Design review of the part built by this model. Coordinates are the model's own, in mm. A direction names the side the tool comes from. Give positions to 0.01 mm unless a question says otherwise; leave off trailing zeros. Loops run counter-clockwise (first coordinate to the right, second up) from the corner with the lowest first, then second, coordinate; pieces in that order, holes last. Notation, with made-up numbers: M 41,49.25 L 90,49.25 A20 cw 90,78.25 Z; hole C 58,85.25 d8. An arc over 180 degrees is marked long. Answer as CSV lines item,"result".
```python
from build123d import *

# Parameters (mm, degrees)
SKETCH1_W           = 38.1
SKETCH1_H           = 10.16
SKETCH1_W_2         = 12.7
SKETCH1_R           = 2.54
BOSS_EXTRUDE1_DEPTH = 50.8
SKETCH2_W           = 63.5
SKETCH2_H           = 50.8
CUT_EXTRUDE1_DEPTH  = 61.761238467


with BuildPart() as part:
    # Sketch1 → Boss-Extrude1 (new body)
    # profile 1 of 3: a face of its own
    with BuildSketch(Plane(origin=(0, 0, 0), x_dir=(1, 0, 0), z_dir=(0, 1, 0))):
        with Locations((0, -1.905)):
            Rectangle(SKETCH1_W, SKETCH1_H)
    # profile 2 of 3: a face of its own
    with BuildSketch(Plane(origin=(0, 0, 0), x_dir=(1, 0, 0), z_dir=(0, 1, 0))):
        with Locations((-25.4, -1.905)):
            Rectangle(SKETCH1_W_2, SKETCH1_H)
        with Locations(Location((-25.4, -1.905, 0), (0, 0, 270))):
            Circle(SKETCH1_R, mode=Mode.SUBTRACT)
    # profile 3 of 3: a face of its own
    with BuildSketch(Plane(origin=(0, 0, 0), x_dir=(1, 0, 0), z_dir=(0, 1, 0))):
        with Locations((25.4, -1.905)):
            Rectangle(SKETCH1_W_2, SKETCH1_H)
        with Locations(Location((25.4, -1.905, 0), (0, 0, 270))):
            Circle(SKETCH1_R, mode=Mode.SUBTRACT)
    extrude(amount=BOSS_EXTRUDE1_DEPTH)

    # Sketch2 → Cut-Extrude1 (cut, through all)
    # profile 1 of 2: a face of its own
    with BuildSketch(Plane.XY.offset(6.985)):
        with Locations((0, 25.4)):
            Rectangle(SKETCH2_W, SKETCH2_H)
        with BuildLine():
            Line((-11.43, 10.16), (-30.48, 10.16))
            Line((-30.48, 10.16), (-30.48, 14.258420741))
            Line((-30.48, 14.258420741), (-18.493061175, 14.258420741))
            ThreePointArc((-18.493061175, 14.258420741), (0, 46.99), (18.493061175, 14.258420741))
            Line((18.493061175, 14.258420741), (30.48, 14.258420741))
            Line((30.48, 14.258420741), (30.48, 10.16))
            Line((30.48, 10.16), (11.43, 10.16))
            ThreePointArc((11.43, 10.16), (0, 44.45), (-11.43, 10.16))
        make_face(mode=Mode.SUBTRACT)
    # profile 2 of 2: a face of its own
    with BuildSketch(Plane.XY.offset(6.985)):
        with Locations((0, 25.4)):
            Rectangle(SKETCH2_W, SKETCH2_H)
        with BuildLine():
            Line((-11.43, 10.16), (-30.48, 10.16))
            Line((-30.48, 10.16), (-30.48, 14.258420741))
            Line((-30.48, 14.258420741), (-18.493061175, 14.258420741))
            ThreePointArc((-18.493061175, 14.258420741), (0, 46.99), (18.493061175, 14.258420741))
            Line((18.493061175, 14.258420741), (30.48, 14.258420741))
            Line((30.48, 14.258420741), (30.48, 10.16))
            Line((30.48, 10.16), (11.43, 10.16))
            ThreePointArc((11.43, 10.16), (0, 44.45), (-11.43, 10.16))
        make_face(mode=Mode.SUBTRACT)
    extrude(amount=-CUT_EXTRUDE1_DEPTH, mode=Mode.SUBTRACT)


solid = part.part
```
1. To check wall thickness, follow L1, parallel to Z at x = 25.4, y = 11.85 (3 decimals); L2, parallel to X at y = 25.4, z = 4.5; L3, parallel to X at y = 13, z = -2.5. State the ranges of each line that lie inside material, in increasing order. Write a range as [from, to].
Answer block:
L1,"[-3.175, -0.635], [4.445, 6.985]"
L2,"[-21.59, -19.05], [19.05, 21.59]"
L3,"[-30.48, -14.46], [14.46, 30.48]"
2. The part is to be moulded in two halves that separate along Y. For faces 3 (the cylindrical face through (-27.88, 12.18, 1.35)), 4 (the flat face through (22, 14.258, 2)), 5 (the flat face through (21, 10.16, 2)), say which applies: pulls with the +Y half, pulls with the -Y half, needs draft (parallel to the pull), parting line crosses it, or undercut.
Answer block:
face 3,"needs draft"
face 4,"undercut"
face 5,"pulls with the -Y half"
3. We need section B-B, the plane x = 25.4. Write out the cut boundary in (y, z) (3 decimals), plus the area to 3 significant figures.
Answer block:
outline,"M 10.16,-3.175 L 14.258,-3.175 L 14.258,-0.635 L 10.16,-0.635 Z; M 10.16,4.445 L 14.258,4.445 L 14.258,6.985 L 10.16,6.985 Z"
area,"20.8 mm²"
4. For faces 1 (the flat face through (30.48, 12, 2)), 2 (the flat face through (-22, 14.258, 2)), list the 3-axis set-ups (+Z, -Z, +X, -X, +Y, -Y) from which the entire face can be reached by the end or side of a thin tool; tool diameter is ignored.
Answer block:
face 1,"+Z, -Z, +X, +Y, -Y"
face 2,"+Z, -Z, -X"
5. We need section C-C, the plane z = 0.5. Write out the cut boundary in (x, y).
Answer block:
outline,"M -30.48,10.16 L -27.52,10.16 L -27.52,14.26 L -30.48,14.26 Z; M -23.28,10.16 L -11.43,10.16 A19.05 cw long 11.43,10.16 L 23.28,10.16 L 23.28,14.26 L 18.49,14.26 A21.59 ccw long -18.49,14.26 L -23.28,14.26 Z; M 27.52,10.16 L 30.48,10.16 L 30.48,14.26 L 27.52,14.26 Z"
6. For P1, Ø5, axis at y = 19, z = -1.5, coming from the -X side; P2, Ø1.5, axis at y = 35, z = 1.5, coming from the -X side; P3, Ø1, axis at x = -9.5, z = -2, coming from the -Y side, all flat-tipped, find the tip position at first contact; note any pin that passes through.
Answer block:
P1,"x = -21.23"
P2,"x = -19.69"
P3,"y = 41.61"
7. We need section D-D, the plane z = -2.5. Write out the cut boundary in (x, y).
Answer block:
outline,"M -30.48,10.16 L -11.43,10.16 A19.05 cw long 11.43,10.16 L 30.48,10.16 L 30.48,14.26 L 18.49,14.26 A21.59 ccw long -18.49,14.26 L -30.48,14.26 Z"
8. We need section A-A, the plane y = 25.4. Write out the cut boundary in (x, z) (3 decimals).
Answer block:
outline,"M -21.59,-3.175 L -19.05,-3.175 L -19.05,6.985 L -21.59,6.985 Z; M 19.05,-3.175 L 21.59,-3.175 L 21.59,6.985 L 19.05,6.985 Z"
